Check sheet for the modelled part. Datum: model origin and axes. Units: mm. A direction names the side the tool comes from. Coordinates: 2 decimals unless noted, no trailing zeros. Loops run counter-clockwise (first coordinate to the right, second up) from the corner with the lowest first, then second, coordinate; pieces in that order, holes last.
```python
from build123d import *

# Parameters (mm, degrees)
EXTRUDE1_DEPTH = 45


with BuildPart() as part:
    # Sketch1 → Extrude1 (new body)
    with BuildSketch(Plane.XY):
        with BuildLine():
            Line((-95, 40), (49, 40))
            ThreePointArc((49, 40), (55.44932167, 42.08898154), (59.449095356, 47.5625))
            ThreePointArc((59.449095356, 47.5625), (61.267174304, 50.050462937), (64.198684154, 51))
            Line((64.198684154, 51), (95, 51))
            ThreePointArc((95, 51), (98.535533906, 49.535533906), (100, 46))
            Line((100, 46), (100, -35))
            ThreePointArc((100, -35), (98.535533906, -38.535533906), (95, -40))
            Line((95, -40), (-95, -40))
            ThreePointArc((-95, -40), (-98.535533906, -38.535533906), (-100, -35))
            Line((-100, -35), (-100, 35))
            ThreePointArc((-100, 35), (-98.535533906, 38.535533906), (-95, 40))
        make_face()
    extrude(amount=EXTRUDE1_DEPTH)


solid = part.part
```
1) Depth check by flat-ended pin: pin 1 (6 mm diameter, centred on x = -58, z = 35.5, fed in from +Y); pin 2 (12 mm diameter, centred on x = -36.5, y = 16, fed in from -Z); pin 3 (10 mm diameter, centred on x = 46.5, z = 40, fed in from +Y). Enter the tip coordinate at first touch or a pass-through.
Answer sheet:
pin 1: stops at y = 40
pin 2: stops at z = 0
pin 3: stops at y = 40.29
2) Section check A-A on z = 7. Enter the section's corners in (x, y), plus the area to 3 significant figures.
Answer sheet:
outline: (-100, -35) arc R5 ccw to (-95, -40) - (95, -40) arc R5 ccw to (100, -35) - (100, 46) arc R5 ccw to (95, 51) - (64.2, 51) arc R5 ccw to (59.45, 47.56) arc R11 cw to (49, 40) - (-95, 40) arc R5 ccw to (-100, 35) - close
area: 16,400 mm2
3) Set-up check for faces 1 (the cylindrical face through (99, -38, 22)), 2 (the flat face through (-24, 40, 22)): record each of +Z, -Z, +X, -X, +Y, -Y from which the full face is reachable in a straight line by a thin tool's end or side.
Answer sheet:
face 1: +Z, -Z, +X, -Y
face 2: +Z, -Z, -X, +Y
4) Section check B-B on x = -41.5. Enter the section's corners in (y, z), plus the area to 3 significant figures.
Answer sheet:
outline: (-40, 0) - (40, 0) - (40, 45) - (-40, 45) - close
area: 3,600 mm2
5) Scan lines: line 1 (Y direction, x = 19, z = 29); line 2 (Y direction, x = 58, z = 14); line 3 (X direction, y = 38, z = 3.5). Record each from-to range of solid material in increasing order.
Answer sheet:
line 1: y = -40 to 40
line 2: y = -40 to 44.68
line 3: x = -99 to 100
